```python
from build123d import *

# Parameters (mm, degrees)
CHAMFER2_SIZE      = 0.254
CHAMFER3_SIZE      = 0.508
SKETCH4_R          = 1.89865
CUT_EXTRUDE1_DEPTH = 5.08


with BuildPart() as part:
    # Sketch1 → Revolve1 (revolve)
    with BuildSketch(Plane.XY, mode=Mode.PRIVATE) as revolve1_sk:
        with BuildLine():
            Line((0, 5.55625), (4.365625, 5.55625))
            Line((4.365625, 5.55625), (4.365625, 0))
            Line((4.365625, 0), (13.17625, 0))
            Line((13.17625, 0), (15.24, -2.06375))
            Line((15.24, -2.06375), (25.4, -2.06375))
            Line((25.4, -2.06375), (25.4, 5.55625))
            ThreePointArc((25.4, 5.55625), (12.951509565, 9.353797823), (0, 10.63625))
            Line((0, 10.63625), (0, 5.55625))
        make_face()
    revolve(revolve1_sk.sketch.rotate(Axis((0, 18.150046132, 0), (0, -1, 0)), 90), axis=Axis((0, 18.150046132, 0), (0, -1, 0)))

    # Chamfer2
    chamfer2_edges = [part.edges().sort_by_distance(p)[0] for p in [
        (0, -2.06375, -25.4),
    ]]
    chamfer(chamfer2_edges, length=CHAMFER2_SIZE)

    # Chamfer3
    # the kernel refuses this chamfer: 0.943428571, 0.508 mm, written as the material it takes off along each edge
    with BuildSketch(Plane(origin=(0, 5.55625, 0), x_dir=(0, 0, 1), z_dir=(1, 0, 0))) as chamfer3_piece_1:
        with BuildLine():
            Line((25.4, CHAMFER3_SIZE), (24.541242074, -0.350757926))
            ThreePointArc((24.541242074, -0.350757926), (24.955132553, -0.183462114), (25.4, 0))
            Line((25.4, 0), (25.4, CHAMFER3_SIZE))
        make_face()
    revolve(axis=Axis((0, 5.55625, 0), (0, -1, 0)), mode=Mode.SUBTRACT)

    # Sketch4 → Cut-Extrude1 (cut)
    with BuildSketch(Plane.XZ.offset(2.06375)):
        with Locations(Location((19.05, 0, 0), (0, 0, 270))):
            Circle(SKETCH4_R)
        with Locations(Location((-9.525, 16.497783942, 0), (0, 0, 270))):
            Circle(SKETCH4_R)
        with Locations(Location((-9.525, -16.497783942, 0), (0, 0, 90))):
            Circle(SKETCH4_R)
    extrude(amount=-CUT_EXTRUDE1_DEPTH, mode=Mode.SUBTRACT)


solid = part.part
```
The model under review builds one solid part; all positions refer to its coordinate system, in mm. Round coordinates to 2 decimals unless told otherwise and drop trailing zeros. Write each loop counter-clockwise with the first axis right and the second up, starting at its lowest first coordinate (ties: lowest second). Pieces come first, ordered by that corner, then holes. Notation, with made-up numbers: (30, 42.5) - (52, 42.5) arc R23 cw to (52, 58.5) - close; hole circle Ø10 at (-7.75, -22). An arc over 180 degrees is marked (long way). Answer as CSV lines item,"result". Start each with the question number.
(1) For pin 1 Ø2.5 at (x, z) = (-1, -1.5) entering from -Y; pin 2 Ø1.1 at (x, z) = (-10, 17) entering from -Y; pin 3 Ø1.5 at (x, z) = (16.5, 8) entering from +Y, all flat-tipped, find the tip position at first contact; note any pin that passes through.
(2) We need section C-C on y = 4. State the section outline as (x, z) points.
(3) We need section D-D on y = -1. Give the number of separate pieces and of enclosed holes in the cut face, plus the area to 3 significant figures.
(4) We need section A-A on x = 0. State the section outline as (y, z) points, plus the area to 3 significant figures.
(5) Draft analysis for pull direction X (two halves, no side actions). For faces 1 (the cylindrical face through (-9.608, 0.441, -18.395)), 2 (the flat face through (11, -2.064, -11)), 3 (the cylindrical face through (15.456, 1.667, -20.157)), state which applies: pulls with the +X half, pulls with the -X half, needs draft (parallel to the pull), parting line crosses it, or undercut.
(6) To check wall thickness, follow line 1 (X direction, y = 0.5, z = 0); line 2 (X direction, y = 3.25, z = 0); line 3 (X direction, y = 2.25, z = -1). State the ranges of each line that lie inside material, in increasing order.
(7) We need section B-B on z = 0. State the section outline as (x, y) points.
Worked answers:
1,pin 1,"y = 5.56"
1,pin 2,"y = 3.02"
1,pin 3,"y = 8.25"
2,outline,"circle Ø50.8 at (0, 0); hole circle Ø8.73 at (0, 0)"
3,separate pieces,"1"
3,enclosed holes,"4"
3,area,"1,360 mm²"
4,outline,"(-2.06, -25.15) - (-1.81, -25.4) - (5.05, -25.4) - (5.91, -24.54) arc R66.04 ccw to (5.91, 24.54) - (5.05, 25.4) - (-1.81, 25.4) - (-2.06, 25.15) - (-2.06, 15.24) - (0, 13.18) - (0, 4.37) - (5.56, 4.37) - (5.56, -4.37) - (0, -4.37) - (0, -13.18) - (-2.06, -15.24) - close"
4,area,"453 mm²"
5,face 1,"undercut"
5,face 2,"needs draft"
5,face 3,"parting line crosses it"
6,line 1,"-25.4 to -4.37, 4.37 to 17.15, 20.95 to 25.4"
6,line 2,"-25.4 to -4.37, 4.37 to 25.4"
6,line 3,"-25.38 to -4.25, 4.25 to 17.44, 20.66 to 25.38"
7,outline,"(-25.4, -1.81) - (-25.15, -2.06) - (-15.24, -2.06) - (-13.18, 0) - (-4.37, 0) - (-4.37, 5.56) - (4.37, 5.56) - (4.37, 0) - (13.18, 0) - (15.24, -2.06) - (17.15, -2.06) - (17.15, 3.02) - (20.95, 3.02) - (20.95, -2.06) - (25.15, -2.06) - (25.4, -1.81) - (25.4, 5.05) - (24.54, 5.91) arc R66.04 ccw to (-24.54, 5.91) - (-25.4, 5.05) - close"
